Geometry: see drawing. Coordinates: mm, zero at the bounding-box minimum. Round coordinates to 2 decimals unless told otherwise and drop trailing zeros. Loops run counter-clockwise (first coordinate to the right, second up) from the corner with the lowest first, then second, coordinate; pieces in that order, holes last. Notation, with made-up numbers: (24, -6) - (39, -6) arc R12 ccw to (39, 9) - close; hole circle Ø9 at (-39.75, 32). An arc over 180 degrees is marked (long way). Answer in a Markdown table with one row per item. Add a question column.
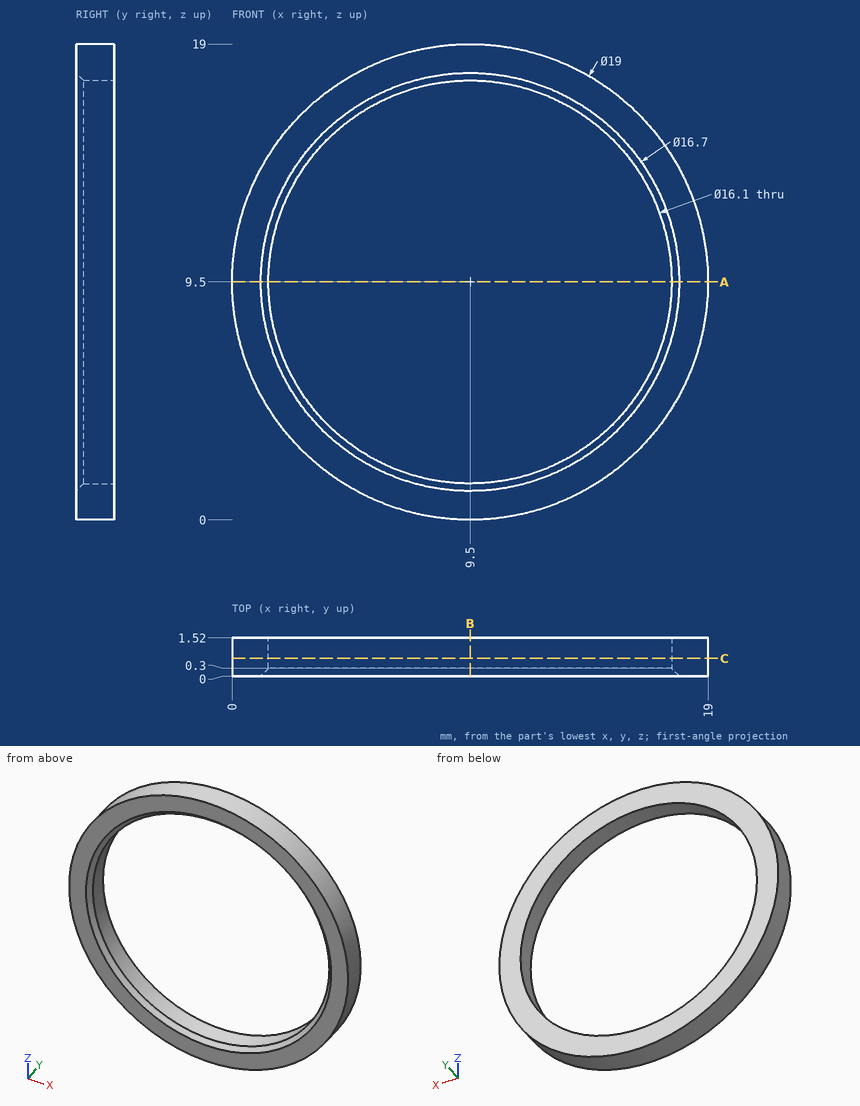
1) Section A-A, the plane z = 9.5. Return the cut outline in (x, y).
2) Section B-B, the plane x = 9.5. Return the cut outline in (y, z), and give its area (3 significant figures).
3) Section C-C, the plane y = 0.7. Return the cut outline in (x, z).
4) Material intervals for line 1 along X through (y, z) = (0.9, 9.5); line 2 along Z through (x, y) = (16.25, 0.65), sorted ascending. Write a range as from..to.
Evaluation:
| question | item | result |
|---|---|---|
| 1 | outline | (0, 0) - (1.15, 0) - (1.45, 0.3) - (1.45, 1.52) - (0, 1.52) - close; (17.55, 0.3) - (17.85, 0) - (19, 0) - (19, 1.52) - (17.55, 1.52) - close |
| 2 | outline | (0, 0) - (1.52, 0) - (1.52, 1.45) - (0.3, 1.45) - (0, 1.15) - close; (0, 17.85) - (0.3, 17.55) - (1.52, 17.55) - (1.52, 19) - (0, 19) - close |
| 2 | area | 4.32 mm² |
| 3 | outline | circle Ø19 at (9.5, 9.5); hole circle Ø16.1 at (9.5, 9.5) |
| 4 | line 1 | x = 0..1.45, 17.55..19 |
| 4 | line 2 | z = 2.82..5.11, 13.89..16.18 |
